```python
from build123d import *

# Parameters (mm, degrees)
SKETCH2_W           = 101.6
SKETCH2_H           = 50.8
BOSS_EXTRUDE1_DEPTH = 3
FILLET1_R           = 25.4
SKETCH4_W           = 25.4
SKETCH4_H           = 3
CUT_EXTRUDE1_DEPTH  = 3
SKETCH6_W           = 50.8
SKETCH6_H           = 12.7
CUT_EXTRUDE2_DEPTH  = 10
FILLET2_R           = 6


with BuildPart() as part:
    # Sketch2 → Boss-Extrude1 (new body)
    with BuildSketch(Plane(origin=(0, 0, 0), x_dir=(0, 0, -1), z_dir=(1, 0, 0))):
        with Locations((50.8, 25.4)):
            Rectangle(SKETCH2_W, SKETCH2_H)
    extrude(amount=BOSS_EXTRUDE1_DEPTH)

    # Fillet1
    fillet1_edges = [part.edges().sort_by_distance(p)[0] for p in [
        (1.5, 50.8, 0),
        (1.5, 50.8, -101.6),
    ]]
    fillet(fillet1_edges, radius=FILLET1_R)

    # Sketch4 → Cut-Extrude1 (cut)
    with BuildSketch(Plane(origin=(3, 0, 0), x_dir=(0, 0, -1), z_dir=(1, 0, 0))):
        with Locations((12.7, 1.5)):
            Rectangle(SKETCH4_W, SKETCH4_H)
        with Locations((88.9, 1.5)):
            Rectangle(SKETCH4_W, SKETCH4_H)
    extrude(amount=-CUT_EXTRUDE1_DEPTH, mode=Mode.SUBTRACT)

    # Sketch6 → Cut-Extrude2 (cut)
    with BuildSketch(Plane(origin=(3, 0, 0), x_dir=(0, 0, -1), z_dir=(1, 0, 0))):
        with Locations((50.8, 28.4)):
            Rectangle(SKETCH6_W, SKETCH6_H)
    extrude(amount=-CUT_EXTRUDE2_DEPTH, mode=Mode.SUBTRACT)

    # Fillet2
    fillet2_edges = [part.edges().sort_by_distance(p)[0] for p in [
        (1.5, 22.05, -25.4),
        (1.5, 34.75, -25.4),
        (1.5, 34.75, -76.2),
        (1.5, 22.05, -76.2),
    ]]
    fillet(fillet2_edges, radius=FILLET2_R)


solid = part.part
```
Check sheet for the modelled part. Datum: model origin and axes. Units: mm. A direction names the side the tool comes from. Round coordinates to 2 decimals unless told otherwise and drop trailing zeros. Write each loop counter-clockwise with the first axis right and the second up, starting at its lowest first coordinate (ties: lowest second). Pieces come first, ordered by that corner, then holes. Notation, with made-up numbers: (65.25, 66.5) -> (122.25, 66.5) arc R20 ccw to (122.25, 74.5) -> close; hole circle Ø11 at (78, -6). An arc over 180 degrees is marked (long way). One line per question, with ' | ' between items. Start each with the question number.
1. Release check for a two-part mould opening along Z. For faces 6 (the face through (0, 20, -50)), 7 (the face through (1.479, 23.761, -74.396)), 8 (the face through (1, 14, -101.6)) record: +Z half, -Z half, draft (parallel to the pull), parting line (faces both ways), or undercut.
2. Sectioned sample at C-C, the plane z = -73. Record the cut outline in (x, y).
3. Depth check by flat-ended pin: pin 1 (0.9 mm diameter, centred on x = 1.5, y = 1.5, fed in from +Z); pin 2 (1.5 mm diameter, centred on x = 1.5, z = -91.5, fed in from -Y). Enter the tip coordinate at first touch or a pass-through.
4. Sectioned sample at D-D, the plane y = 42. Record the cut outline in (x, z), then the cut area to 3 significant figures.
5. Sectioned sample at B-B, the plane x = 0.75. Record the cut outline in (y, z).
6. Set-up check for faces 1 (the face through (1, 0, -50)), 2 (the face through (1.479, 32.946, -74.489)), 3 (the face through (2, 3, -13)), 4 (the face through (1, 50.8, -50)), 5 (the face through (2, 1, -76.2)): record each of +Z, -Z, +X, -X, +Y, -Y from which the full face is reachable in a straight line by a thin tool's end or side.
7. Sectioned sample at A-A, the plane z = -54.5. Record the cut outline in (x, y), then the cut area to 3 significant figures.
8. Scan lines: line 1 along Y through (x, z) = (2, -41.5); line 2 along Z through (x, y) = (2.55, 23); line 3 along Y through (x, z) = (2.05, -73). Record each from-to range of solid material in increasing order. Write a range as from..to.
Taken from the geometry:
1) face 6: draft | face 7: undercut | face 8: -Z half
2) outline: (0, 0) -> (3, 0) -> (3, 22.74) -> (0, 22.74) -> close; (0, 34.06) -> (3, 34.06) -> (3, 50.8) -> (0, 50.8) -> close
3) pin 1: stops at z = -25.4 | pin 2: stops at y = 3
4) outline: (0, -95.42) -> (3, -95.42) -> (3, -6.18) -> (0, -6.18) -> close | area: 268 mm^2
5) outline: (0, -76.2) -> (3, -76.2) -> (3, -101.6) -> (25.4, -101.6) arc R25.4 ccw to (50.8, -76.2) -> (50.8, -25.4) arc R25.4 ccw to (25.4, 0) -> (3, 0) -> (3, -25.4) -> (0, -25.4) -> close; hole (22.05, -70.2) arc R6 ccw to (28.05, -76.2) -> (28.75, -76.2) arc R6 ccw to (34.75, -70.2) -> (34.75, -31.4) arc R6 ccw to (28.75, -25.4) -> (28.05, -25.4) arc R6 ccw to (22.05, -31.4) -> close
6) face 1: +Z, -Z, +X, -X, -Y | face 2: +X, -X | face 3: +Z, +X, -X, -Y | face 4: +Z, -Z, +X, -X, +Y | face 5: -Z, +X, -X, -Y
7) outline: (0, 0) -> (3, 0) -> (3, 22.05) -> (0, 22.05) -> close; (0, 34.75) -> (3, 34.75) -> (3, 50.8) -> (0, 50.8) -> close | area: 114 mm^2
8) line 1: y = 0..22.05, 34.75..50.8 | line 2: z = -101.6..-73.44, -28.16..0 | line 3: y = 0..22.74, 34.06..50.8
